Build history of the part. All positions in model axes, mm. Give positions to 0.01 mm unless a question says otherwise; leave off trailing zeros. Order: outer loops, then holes, each group sorted by start corner. A loop starts at its lowest first (then second) coordinate and runs counter-clockwise, first axis right, second up. Notation, with made-up numbers: M -29.5,27 L -9.5,27 A32 cw -9.5,64 Z; hole C 55.5,76 d7. An arc over 180 degrees is marked long. Use CSV: the item, a comma, the result in double quotes. Start each with the question number.
Item 1: Pin check, flat tips, straight feed: P1, Ø1.6, axis at y = 52, z = 1, coming from the -X side; P2, Ø1, axis at x = 190.5, z = 1, coming from the -Y side; P3, Ø1, axis at y = -1, z = 1, coming from the +X side. Stop position of each tip, or through.
Item 2: Band-saw the part on B-B on x = 263. Write the cut outline in (y, z) (3 decimals), plus the area to 3 significant figures.
Item 3: Band-saw the part on A-A on y = 7.5. Write the cut outline in (x, z) (3 decimals), plus the area to 3 significant figures.
Item 4: Wall check: line 1 along X through (y, z) = (4.5, 0.65); line 2 along Y through (x, z) = (87, 1.7). Give the ranges that are in metal, low to high.
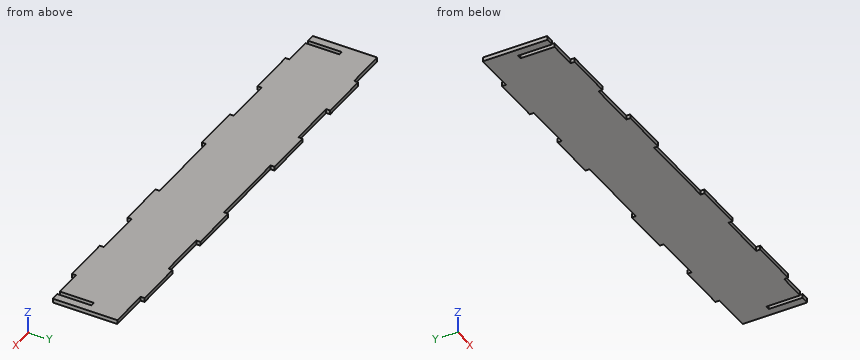
from build123d import *

# Parameters (mm, degrees)
SKETCH1_W               = 355.6
SKETCH1_H               = 50.8
BOSS_EXTRUDE1_DEPTH     = 3.175
SKETCH2_W               = 38.1
SKETCH2_H               = 3.175
BOSS_EXTRUDE2_DEPTH     = 3.175
MIRROR2_COPY_1_SKETCH_W = 38.1
MIRROR2_COPY_1_SKETCH_H = 3.175
MIRROR2_COPY_1_DEPTH    = 3.175
SKETCH3_W               = 3.302
SKETCH3_H               = 26.67
CUT_EXTRUDE1_DEPTH      = 3.175


with BuildPart() as part:
    # Sketch1 → Boss-Extrude1 (new body)
    with BuildSketch(Plane.XY):
        with Locations((177.8, 25.4)):
            Rectangle(SKETCH1_W, SKETCH1_H)
    extrude(amount=BOSS_EXTRUDE1_DEPTH)

    # Sketch2 → Boss-Extrude2 (add)
    with BuildSketch(Plane(origin=(0, 50.8, 0), x_dir=(1, 0, 0), z_dir=(0, 1, 0))):
        with Locations((50.8, -1.5875)):
            Rectangle(SKETCH2_W, SKETCH2_H)
        with Locations((127, -1.5875)):
            Rectangle(SKETCH2_W, SKETCH2_H)
    boss_extrude2 = extrude(amount=BOSS_EXTRUDE2_DEPTH)

    # Mirror1: Boss-Extrude2 across plane
    add(boss_extrude2.mirror(Plane.ZY.offset(-177.8)))

    # Mirror2: Boss-Extrude2 across plane
    add(boss_extrude2.mirror(Plane.ZX.offset(25.4)))

    # Mirror2 copy 1 sketch → Mirror2 copy 1 (add)
    with BuildSketch(Plane(origin=(355.6, 0, 0), x_dir=(-1, 0, 0), z_dir=(0, -1, 0))):
        with Locations((50.8, -1.5875)):
            Rectangle(MIRROR2_COPY_1_SKETCH_W, MIRROR2_COPY_1_SKETCH_H)
        with Locations((127, -1.5875)):
            Rectangle(MIRROR2_COPY_1_SKETCH_W, MIRROR2_COPY_1_SKETCH_H)
    extrude(amount=MIRROR2_COPY_1_DEPTH)

    # Sketch3 → Cut-Extrude1 (cut)
    with BuildSketch(Plane(origin=(0, 0, 0), x_dir=(-1, 0, 0), z_dir=(0, 0, -1))):
        with Locations((-8.001, 13.335)):
            Rectangle(SKETCH3_W, SKETCH3_H)
    cut_extrude1 = extrude(amount=-CUT_EXTRUDE1_DEPTH, mode=Mode.SUBTRACT)

    # Mirror3: Cut-Extrude1 across plane
    add(cut_extrude1.mirror(Plane.ZY.offset(-177.8)), mode=Mode.SUBTRACT)


solid = part.part
Model answer:
1,P1,"stops at x = 31.75"
1,P2,"stops at y = 0"
1,P3,"stops at x = 323.85"
2,outline,"M 0,0 L 50.8,0 L 50.8,3.175 L 0,3.175 Z"
2,area,"161 mm^2"
3,outline,"M 0,0 L 6.35,0 L 6.35,3.175 L 0,3.175 Z; M 9.652,0 L 345.948,0 L 345.948,3.175 L 9.652,3.175 Z; M 349.25,0 L 355.6,0 L 355.6,3.175 L 349.25,3.175 Z"
3,area,"1,110 mm^2"
4,line 1,"x = 0 to 6.35, 9.65 to 345.95, 349.25 to 355.6"
4,line 2,"y = 0 to 50.8"
